Check sheet for the modelled part. Datum: model origin and axes. Units: mm. Round coordinates to 2 decimals unless told otherwise and drop trailing zeros. Loops run counter-clockwise (first coordinate to the right, second up) from the corner with the lowest first, then second, coordinate; pieces in that order, holes last. Notation, with made-up numbers: (56.5, -12) - (108.5, -12) arc R20 ccw to (108.5, 16) - close; hole circle Ø6 at (67, -2). An arc over 180 degrees is marked (long way). Answer in a Markdown table with one row per item. Add a question column.
(1) Cross-section at B-B on x = 2.05. Enter the section's corners in (y, z), then the cut area to 3 significant figures.
(2) Cross-section at D-D on y = -8. Enter the section's corners in (x, z).
(3) Cross-section at A-A on y = -2.25. Enter the section's corners in (x, z).
(4) Gauge pin test, flat end, axial feed: pin 1 (1.6 mm diameter, centred on y = -2.91, z = 17.27, fed in from -X). Record the tip position at first contact, or that the pin passes through.
(5) Cross-section at C-C on z = 24.5. Enter the section's corners in (x, y).
(6) Thickness scan on line 1 along Y through (x, z) = (1.8, 19); line 2 along Z through (x, y) = (1.5, -5.5); line 3 along Z through (x, y) = (2.3, 2.5). Record the ranges inside material, lowest first.
Autodesk Inventor part; units mm, degrees
ref_plane "YZ Plane" through (0, 0, 0) normal (1, 0, 0) x (0, 1, 0)
ref_plane "XZ Plane" through (0, 0, 0) normal (0, 1, 0) x (-1, 0, 0)
ref_plane "XY Plane" through (0, 0, 0) normal (0, 0, 1) x (1, 0, 0)
sketch "スケッチ1" plane through (0, 0, 0) normal (1, 0, 0) x (0, 1, 0)
  line L0 (7.087, 17.2652) -> (-12.913, 17.2652)
  line L1 (-12.913, 17.2652) -> (-12.913, -4.7348)
  line L2 (-12.913, -4.7348) -> (7.087, -4.7348)
  line L3 (7.087, -4.7348) -> (7.087, 17.2652)
  arc A0 (7.087, 17.2652) -> (-12.913, 17.2652) centre (-2.913, 17.2652) ccw
  point P0 (0, 0)
  dimension "d0" = 20
  dimension "d1" = 22
extrude "押し出し1" add sketch "スケッチ1" along normal blind 3
sketch "スケッチ2" plane through (3, 0, 0) normal (1, 0, 0) x (0, 0, -1)
  arc A0 (-17.2652, 7.087) -> (-17.2652, -12.913) centre (-17.2652, -2.913) ccw
  circle A1 centre (-17.2652, -2.913) radius 1
  point P0 (0, 0)
  dimension "d4" = 2
hole "穴1" at (3, -2.913, 17.2652) direction (-1, 0, 0) diameter 2 depth 10
equation "\"BendRadius\" = Thickness"
equation "\"BendReliefWidth\" = Thickness"
equation "\"BendReliefDepth\" = 0.5 * Thickness"
equation "\"CornerReliefSize\" = 4 * Thickness"
equation "\"MinimumRemnant\" = 2 * Thickness"
equation "\"TransitionRadius\" = BendRadius"
equation "\"JacobiRadiusSize\" = BendRadius"
equation "\"GapSize\" = Thickness"
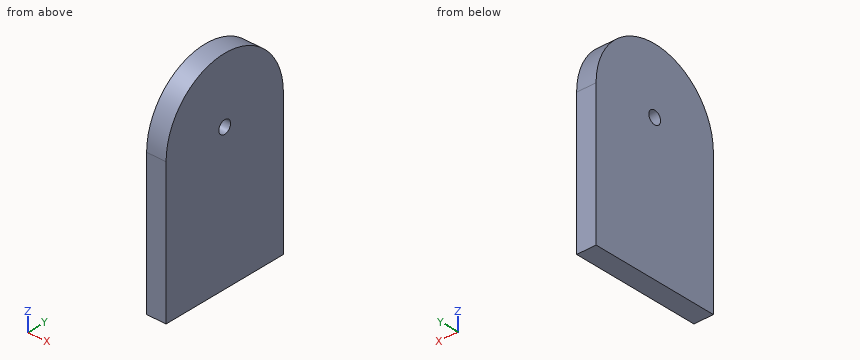
Answers:
| question | item | result |
|---|---|---|
| 1 | outline | (-12.91, -4.73) - (7.09, -4.73) - (7.09, 17.27) arc R10 ccw to (-12.91, 17.27) - close; hole circle Ø2 at (-2.91, 17.27) |
| 1 | area | 594 mm^2 |
| 2 | outline | (0, -4.73) - (3, -4.73) - (3, 25.87) - (0, 25.87) - close |
| 3 | outline | (0, -4.73) - (3, -4.73) - (3, 16.52) - (0, 16.52) - close; (0, 18.01) - (3, 18.01) - (3, 27.24) - (0, 27.24) - close |
| 4 | pin 1 | passes through |
| 5 | outline | (0, -9.82) - (3, -9.82) - (3, 3.99) - (0, 3.99) - close |
| 6 | line 1 | y = -12.76 to 6.94 |
| 6 | line 2 | z = -4.73 to 26.92 |
| 6 | line 3 | z = -4.73 to 25.67 |
